Here's how the part is built. I have some questions about the finished solid (model axes, mm). Face numbers are marked on the shaded views. A direction names the side the tool comes from. Coordinates: 2 decimals unless noted, no trailing zeros. Write each loop counter-clockwise with the first axis right and the second up, starting at its lowest first coordinate (ties: lowest second). Pieces come first, ordered by that corner, then holes. Notation, with made-up numbers: M -27,-16 L -23,-16 A27 ccw -23,11 Z; hole C 69.25,21.25 d11. An arc over 180 degrees is marked long. Use one line per item in the form item = value. Start each with the question number.
1. I want a section at B-B, the plane y = 59. List the corners of the cut face in (x, z) for me (3 decimals).
2. Thinking about a two-plate mould opening in Z: for the marked faces 4, 5 and 6, which applies, released by +Z, released by -Z, zero draft, split by the parting line, or undercut?
3. I'm going to push flat-ended pins straight in: pin 1 Ø1 at (y, z) = (70.5, -68) entering from +X; pin 2 Ø2 at (x, y) = (82.5, 9) entering from +Z; pin 3 Ø8 at (y, z) = (54, -83) entering from +X; pin 4 Ø10 at (x, z) = (167, -67.5) entering from -Y. Where does each tip first touch, or does it pass through?
4. I want a section at D-D, the plane z = -59. Count the separate pieces of the cut face and the enclosed holes in it, plus the area to 3 significant figures.
5. On a 3-axis mill with a long thin cutter (end or side, diameter ignored), from which of +Z, -Z, +X, -X, +Y, -Y can I reach the whole of each face in a straight line? I mean the marked faces 1, 2 and 3. Say none if no direction works.
6. Please list where these lines run through material, in increasing order: line 1 along Y through (x, z) = (155, -67); line 2 along Z through (x, y) = (25, 49); line 3 along Z through (x, y) = (100, 71.5). Write a range as [from, to].
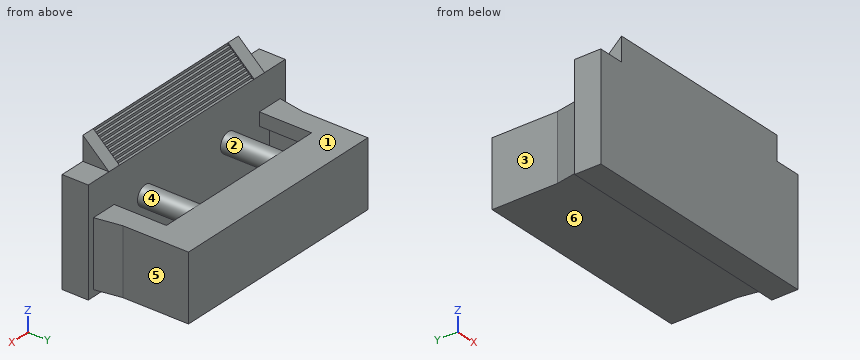
Autodesk Inventor part; units mm, degrees
ref_plane "Work Plane1" through (120.65, 0, -124.6632) normal (1, 0, 0) x (0, 0, -1)
ref_plane "YZ Plane" through (0, 0, 0) normal (1, 0, 0) x (0, 1, 0)
ref_plane "XZ Plane" through (0, 0, 0) normal (0, 1, 0) x (-1, 0, 0)
sketch "Sketch1" plane through (0, 0, 0) normal (0, 1, 0) x (-1, 0, 0)
  line L0 (0, 0) -> (-241.3, 0)
  line L1 (-241.3, 0) -> (-241.3, -124.6632)
  line L2 (-241.3, -124.6632) -> (0, -124.6632)
  line L3 (0, -124.6632) -> (0, 0)
  dimension "d0" = 124.6632
  dimension "d1" = 241.3
extrude "Extrusion1" add sketch "Sketch1" along normal blind 25.4
sketch "Sketch2" plane through (241.3, 0, 0) normal (1, 0, 0) x (0, 0, -1)
  line L0 (124.6632, 0) -> (226.2632, 0) construction
  line L1 (23.0632, 25.4) -> (0, 0)
  line L2 (0, 0) -> (0, 25.4)
  line L3 (0, 0) -> (0, 25.4)
  line L4 (0, 25.4) -> (23.0632, 25.4)
  line L5 (0, 0) -> (23.0632, 0)
  line L6 (0, 0) -> (124.6632, 0)
  line L7 (23.0632, 0) -> (23.0632, 25.4)
extrude "Extrusion2" cut sketch "Sketch2" against normal blind 25.4
ref_plane "Work Plane1" through (120.65, 0, -124.6632) normal (1, 0, 0) x (0, 0, -1)
mirror "Mirror1" about plane through (120.65, 0, -124.6632) normal (1, 0, 0) of "Extrusion2"
extrude "Extrusion3" cut sketch "Sketch2" against normal blind 228.6 contours L1 L2 L4
sketch "Sketch3" plane through (120.65, 0, -124.6632) normal (1, 0, 0) x (0, 0, -1)
  line L0 (-101.6, 25.4) -> (-101.6, 22.86)
  line L1 (-101.6, 0) -> (-101.6, 25.4)
  line L2 (-101.6, 22.86) -> (-104.14, 22.86)
  line L3 (-104.14, 22.86) -> (-104.14, 30.1007)
  line L4 (-104.14, 30.1007) -> (-101.6, 30.1564)
  line L5 (-101.6, 30.1564) -> (-101.6, 25.4)
  point P0 (-124.6632, 0)
  dimension "d10" = 2.54
  dimension "d11" = 2.54
extrude "Extrusion4" cut sketch "Sketch3" along normal mid plane 165.1
pattern_linear "Rectangular Pattern1" count 10 spacing 3.429 along (0, -0.7403, 0.6722) of "Extrusion4"
sketch "Sketch4" plane through (0, 25.4, 0) normal (0, 1, 0) x (1, 0, 0)
  line L0 (6.35, 118.3132) -> (234.95, 118.3132)
  line L1 (234.95, 118.3132) -> (234.95, 54.8132)
  line L2 (6.35, 54.8132) -> (6.35, 118.3132)
  line L3 (241.3, 23.0632) -> (241.3, 124.6632)
  line L4 (0, 124.6632) -> (0, 23.0632)
  line L5 (241.3, 124.6632) -> (0, 124.6632)
  line L6 (222.25, 67.5132) -> (222.25, 111.9632)
  line L7 (222.25, 111.9632) -> (19.05, 111.9632)
  line L8 (19.05, 111.9632) -> (19.05, 67.5132)
  line L9 (234.95, 54.8132) -> (222.25, 54.8132)
  line L10 (19.05, 54.8132) -> (6.35, 54.8132)
  circle A0 centre (69.85, 64.3382) radius 9.525
  circle A1 centre (171.45, 64.3382) radius 9.525
  line L11 (19.05, 54.8132) -> (31.75, 54.8132)
  line L12 (31.75, 54.8132) -> (31.75, 67.5132)
  line L13 (31.75, 67.5132) -> (19.05, 67.5132)
  line L14 (222.25, 54.8132) -> (209.55, 54.8132)
  line L15 (209.55, 54.8132) -> (209.55, 67.5132)
  line L16 (209.55, 67.5132) -> (222.25, 67.5132)
  point P0 (0, 0)
  dimension "d17" = 6.35
  dimension "d18" = 6.35
  dimension "d19" = 6.35
  dimension "d23" = 12.7
  dimension "d24" = 12.7
  dimension "d25" = 6.35
  dimension "d26" = 19.05
  dimension "d27" = 19.05
  dimension "d28" = 9.525
  dimension "d29" = 50.8
  dimension "d39" = 12.7
  dimension "d40" = 12.7
  dimension "d41" = 12.7
  dimension "d42" = 12.7
extrude "Extrusion6" add sketch "Sketch4" along normal blind 25.4
chamfer "Chamfer1" distance 25.4 angle 10 1 edges at (234.95, 50.8, -86.5632) measured on face at (234.95, 33.8667, -97.1465)
chamfer "Chamfer2" distance 25.4 angle 10 1 edges at (6.35, 50.8, -86.5632) measured on face at (6.35, 33.8667, -75.9799)
sketch "Sketch5" plane through (0, 50.8, 0) normal (0, 1, 0) x (1, 0, 0)
  line L0 (10.8287, 54.8132) -> (10.8287, 118.3132)
  line L1 (10.8287, 54.8132) -> (31.75, 54.8132)
  line L2 (19.05, 67.5132) -> (19.05, 111.9632)
  line L3 (19.05, 111.9632) -> (222.25, 111.9632)
  line L4 (222.25, 111.9632) -> (222.25, 67.5132)
  line L5 (209.55, 54.8132) -> (230.4713, 54.8132)
  line L6 (230.4713, 118.3132) -> (230.4713, 54.8132)
  line L7 (230.4713, 118.3132) -> (10.8287, 118.3132)
  circle A0 centre (69.85, 64.3382) radius 9.525
  circle A1 centre (171.45, 64.3382) radius 9.525
  line L8 (31.75, 54.8132) -> (31.75, 67.5132)
  line L9 (31.75, 67.5132) -> (19.05, 67.5132)
  line L10 (222.25, 67.5132) -> (209.55, 67.5132)
  line L11 (209.55, 67.5132) -> (209.55, 54.8132)
  point P0 (0, 0)
extrude "Extrusion7" add sketch "Sketch5" along normal blind 25.4
sketch "Sketch6" plane through (0, 76.2, 0) normal (0, 1, 0) x (1, 0, 0)
  line L0 (10.8287, 118.3132) -> (230.4713, 118.3132)
  line L1 (230.4713, 118.3132) -> (230.4713, 54.8132)
  line L2 (230.4713, 54.8132) -> (10.8287, 54.8132)
  line L3 (10.8287, 54.8132) -> (10.8287, 118.3132)
  point P0 (0, 0)
extrude "Extrusion8" add sketch "Sketch6" along normal blind 38.1
properties part number "Stand"
Answer list:
q1.outline = M 10.829,-118.313 L 230.471,-118.313 L 230.471,-54.813 L 209.55,-54.813 L 209.55,-67.513 L 222.25,-67.513 L 222.25,-111.963 L 19.05,-111.963 L 19.05,-67.513 L 31.75,-67.513 L 31.75,-54.813 L 10.829,-54.813 Z; C 69.85,-64.338 d19.05; C 171.45,-64.338 d19.05
q2.face_4 = undercut
q2.face_5 = zero draft
q2.face_6 = released by -Z
q3.pin_1 = 230.47
q3.pin_2 = -9.23
q3.pin_3 = 230.61
q3.pin_4 = 0
q4.separate_pieces = 1
q4.enclosed_holes = 3
q4.area = 18,300 mm²
q5.face_1 = +Z, +X, -X, +Y
q5.face_2 = none
q5.face_3 = +Z, -Z, -X, +Y
q6.line_1 = [0, 25.4], [76.2, 114.3]
q6.line_2 = [-118.31, -111.96], [-67.51, -54.81]
q6.line_3 = [-118.31, -111.96]
